```python
from build123d import *

# Parameters (mm, degrees)
SKETCH1_W           = 61.542579433
SKETCH1_H           = 85.2804315
SKETCH1_R           = 5
SKETCH1_W_2         = 22.337231555
SKETCH1_H_2         = 13.187695593
SKETCH1_W_3         = 26.375391186
BOSS_EXTRUDE1_DEPTH = 5


with BuildPart() as part:
    # Sketch1 → Boss-Extrude1 (new body)
    with BuildSketch(Plane.XY):
        with Locations((254.240343952, 391.464524612)):
            Rectangle(SKETCH1_W, SKETCH1_H)
        with Locations((231.469054236, 408.546029818)):
            Circle(SKETCH1_R, mode=Mode.SUBTRACT)
        with Locations((246.469054236, 408.546029818)):
            Circle(SKETCH1_R, mode=Mode.SUBTRACT)
        with Locations((261.469054236, 408.546029818)):
            Circle(SKETCH1_R, mode=Mode.SUBTRACT)
        with Locations((276.469054236, 408.546029818)):
            Circle(SKETCH1_R, mode=Mode.SUBTRACT)
        with Locations((231.469054236, 392.046029818)):
            Circle(SKETCH1_R, mode=Mode.SUBTRACT)
        with Locations((246.469054236, 392.046029818)):
            Circle(SKETCH1_R, mode=Mode.SUBTRACT)
        with Locations((261.469054236, 392.046029818)):
            Circle(SKETCH1_R, mode=Mode.SUBTRACT)
        with Locations((276.469054236, 392.046029818)):
            Circle(SKETCH1_R, mode=Mode.SUBTRACT)
        with Locations((231.469054236, 375.546029818)):
            Circle(SKETCH1_R, mode=Mode.SUBTRACT)
        with Locations((246.469054236, 375.546029818)):
            Circle(SKETCH1_R, mode=Mode.SUBTRACT)
        with Locations((261.469054236, 375.546029818)):
            Circle(SKETCH1_R, mode=Mode.SUBTRACT)
        with Locations((276.469054236, 375.546029818)):
            Circle(SKETCH1_R, mode=Mode.SUBTRACT)
        with Locations((240.434189057, 423.994173741)):
            Rectangle(SKETCH1_W_2, SKETCH1_H_2, mode=Mode.SUBTRACT)
        with Locations((271.384348223, 423.994173741)):
            Rectangle(SKETCH1_W_3, SKETCH1_H_2, mode=Mode.SUBTRACT)
        with Locations((238.415109241, 358.934875483)):
            Rectangle(SKETCH1_W_3, SKETCH1_H_2, mode=Mode.SUBTRACT)
        with Locations((271.384348223, 358.934875483)):
            Rectangle(SKETCH1_W_3, SKETCH1_H_2, mode=Mode.SUBTRACT)
    extrude(amount=BOSS_EXTRUDE1_DEPTH)


solid = part.part
```
Verification items for the finished model (mm, model axes). A direction names the side the tool comes from. Round coordinates to 2 decimals unless told otherwise and drop trailing zeros. Write each loop counter-clockwise with the first axis right and the second up, starting at its lowest first coordinate (ties: lowest second). Pieces come first, ordered by that corner, then holes. Notation, with made-up numbers: (2.5, -24.5) - (47.5, -24.5) arc R24 ccw to (47.5, 10.5) - close; hole circle Ø5 at (-20, 83). An arc over 180 degrees is marked (long way). Answer as a JSON object with one key per item and string values. Group by question number.
Q1. Mould release check, pull along Y, two halves, no side actions. Record for faces 3 (the flat face through (254, 392, 0)), 4 (the flat face through (229.266, 424, 2)), 5 (the flat face through (254, 434.105, 2)), 6 (the flat face through (238, 365.529, 2)): released by +Y, released by -Y, zero draft, split by the parting line, or undercut.
Q2. Tool access check on faces 1 (the flat face through (254, 392, 5)), 2 (the flat face through (238, 352.341, 2)). Record the directions out of +Z, -Z, +X, -X, +Y, -Y that give a thin tool (end or side, any length) a straight path to the whole face; none if there is none.
Q3. Section check C-C, the plane x = 273. Enter the section's corners in (y, z).
Q4. Section check A-A, the plane y = 419. Enter the section's corners in (x, z), plus the area to 3 significant figures.
Q5. Section check B-B, the plane x = 239. Enter the section's corners in (y, z), plus the area to 3 significant figures.
Q6. Thickness scan on line 1 (X direction, y = 363.5, z = 4.05); line 2 (X direction, y = 409, z = 4.5); line 3 (Y direction, x = 268.5, z = 4.25). Record the ranges inside material, lowest first.
Q7. Section check D-D, the plane z = 3.9. Give the number of separate pieces and of enclosed holes in the cut face, plus the area to 3 significant figures.
Found:
{
 "1": {"face 3": "zero draft", "face 4": "undercut", "face 5": "released by +Y", "face 6": "undercut"},
 "2": {"face 1": "+Z, +X, -X, +Y, -Y", "face 2": "+Z, -Z"},
 "3": {"outline": "(348.82, 0) - (352.34, 0) - (352.34, 5) - (348.82, 5) - close; (365.53, 0) - (371.95, 0) - (371.95, 5) - (365.53, 5) - close; (379.15, 0) - (388.45, 0) - (388.45, 5) - (379.15, 5) - close; (395.65, 0) - (404.95, 0) - (404.95, 5) - (395.65, 5) - close; (412.15, 0) - (417.4, 0) - (417.4, 5) - (412.15, 5) - close; (430.59, 0) - (434.1, 0) - (434.1, 5) - (430.59, 5) - close"},
 "4": {"outline": "(223.47, 0) - (229.27, 0) - (229.27, 5) - (223.47, 5) - close; (251.6, 0) - (258.2, 0) - (258.2, 5) - (251.6, 5) - close; (284.57, 0) - (285.01, 0) - (285.01, 5) - (284.57, 5) - close", "area": "64.1 mm^2"},
 "5": {"outline": "(348.82, 0) - (352.34, 0) - (352.34, 5) - (348.82, 5) - close; (365.53, 0) - (417.4, 0) - (417.4, 5) - (365.53, 5) - close; (430.59, 0) - (434.1, 0) - (434.1, 5) - (430.59, 5) - close", "area": "295 mm^2"},
 "6": {"line 1": "x = 223.47 to 225.23, 251.6 to 258.2, 284.57 to 285.01", "line 2": "x = 223.47 to 226.49, 236.45 to 241.49, 251.45 to 256.49, 266.45 to 271.49, 281.45 to 285.01", "line 3": "y = 348.82 to 352.34, 365.53 to 417.4, 430.59 to 434.1"},
 "7": {"separate pieces": "1", "enclosed holes": "16", "area": "2,970 mm^2"}
}
